Source: CAD feature listing. Evaluate the final solid. Frame: model axes, mm. Give positions to 0.01 mm unless a question says otherwise; leave off trailing zeros. Order: outer loops, then holes, each group sorted by start corner. A loop starts at its lowest first (then second) coordinate and runs counter-clockwise, first axis right, second up. Notation, with made-up numbers: (59.25, 25.25) - (101.25, 25.25) arc R25 ccw to (101.25, 48.25) - close; hole circle Ø4 at (-5, 70.25). An arc over 180 degrees is marked (long way). Use CSV: the item, a comma, the result in double quotes.
```python
from build123d import *

# Parameters (mm, degrees)
SKETCH1_W           = 38.1
SKETCH1_H           = 190.5
SKETCH1_R           = 14.2875
SKETCH1_R_2         = 2.4892
BOSS_EXTRUDE1_DEPTH = 3.175
FILLET1_R           = 6.35


with BuildPart() as part:
    # Sketch1 → Boss-Extrude1 (new, symmetric)
    with BuildSketch(Plane(origin=(0, 0, 0), x_dir=(1, 0, 0), z_dir=(0, 1, 0))):
        with Locations((0, 57.15)):
            Rectangle(SKETCH1_W, SKETCH1_H)
        with Locations(Location((0, 0, 0), (0, 0, 270))):
            Circle(SKETCH1_R, mode=Mode.SUBTRACT)
        with Locations(Location((0, 114.3, 0), (0, 0, 270))):
            Circle(SKETCH1_R, mode=Mode.SUBTRACT)
        with Locations(Location((-12.7, 146.05, 0), (0, 0, 270))):
            Circle(SKETCH1_R_2, mode=Mode.SUBTRACT)
        with Locations(Location((12.7, 146.05, 0), (0, 0, 270))):
            Circle(SKETCH1_R_2, mode=Mode.SUBTRACT)
        with Locations(Location((-12.7, -31.75, 0), (0, 0, 270))):
            Circle(SKETCH1_R_2, mode=Mode.SUBTRACT)
        with Locations(Location((12.7, -31.75, 0), (0, 0, 270))):
            Circle(SKETCH1_R_2, mode=Mode.SUBTRACT)
    extrude(amount=BOSS_EXTRUDE1_DEPTH, both=True)

    # Fillet1
    fillet1_edges = [part.edges().sort_by_distance(p)[0] for p in [
        (-19.05, 0, -152.4),
        (19.05, 0, -152.4),
        (19.05, 0, 38.1),
        (-19.05, 0, 38.1),
    ]]
    fillet(fillet1_edges, radius=FILLET1_R)


solid = part.part
```
Item 1: Section C-C on x = -2. Return the cut outline in (y, z) (3 decimals), then the cut area to 3 significant figures.
Filled in:
outline,"(-3.175, -152.4) - (3.175, -152.4) - (3.175, -128.447) - (-3.175, -128.447) - close; (-3.175, -100.153) - (3.175, -100.153) - (3.175, -14.147) - (-3.175, -14.147) - close; (-3.175, 14.147) - (3.175, 14.147) - (3.175, 38.1) - (-3.175, 38.1) - close"
area,"850 mm2"
Item 2: Material intervals for line 1 (X direction, y = -0.25, z = -146.05); line 2 (X direction, y = 0, z = -10); line 3 (Z direction, x = -7.5, y = -1), sorted ascending. Write a range as from..to.
Filled in:
line 1,"x = -19.05..-15.19, -10.21..10.21, 15.19..19.05"
line 2,"x = -19.05..-10.2, 10.2..19.05"
line 3,"z = -152.4..-126.46, -102.14..-12.16, 12.16..38.1"
Item 3: Section D-D on x = 17. Return the cut outline in (y, z) (3 decimals), then the cut area to 3 significant figures.
Filled in:
outline,"(-3.175, -150.723) - (3.175, -150.723) - (3.175, 36.423) - (-3.175, 36.423) - close"
area,"1,190 mm2"
Item 4: Section B-B on y = -1.25. Count the separate pieces of the cut face and the enclosed holes in it, then the cut area to 3 significant figures.
Filled in:
separate pieces,"1"
enclosed holes,"6"
area,"5,860 mm2"
Item 5: Mould query, pull axis X, two halves, no side actions, for faces 1 (the cylindrical face through (17.24, 0.04, 36.19)), 2 (the cylindrical face through (-12.591, -0.044, 29.263)), 3 (the flat face through (0, 0, 38.1)). Classes: released by +X, released by -X, zero draft, split by the parting line, or undercut.
Filled in:
face 1,"released by +X"
face 2,"undercut"
face 3,"zero draft"
Item 6: First-contact query: pin 1 (8 mm diameter, centred on x = 12.7, z = -146.05, fed in from -Y) (3 decimals). Flat tip, straight axial feed; report the tip coordinate or a pass-through.
Filled in:
pin 1,"stops at y = -3.175"
